Autodesk Fusion 360 part; units mm, degrees
sketch "Sketch1" plane through (0, 0, 0) normal (0, 1, 0) x (1, 0, 0)
  line L0 (0, 0) -> (0, -155)
  line L1 (-77.5, 0) -> (77.5, 0)
  line L2 (77.5, 0) -> (77.5, -155)
  line L3 (77.5, -155) -> (-77.5, -155)
  line L4 (-77.5, -155) -> (-77.5, 0)
  arc A0 (77.5, 0) -> (-77.5, 0) centre (0, 0) ccw
  line L5 (-20, -155) -> (-20, 0)
  arc A1 (20, 0) -> (-20, 0) centre (0, 0) ccw
  line L6 (20, 0) -> (20, -155)
  line L7 (-87.5, -155) -> (-87.5, 0)
  arc A2 (87.5, 0) -> (-87.5, 0) centre (0, 0) ccw
  line L8 (87.5, 0) -> (87.5, -155)
  line L9 (87.5, -155) -> (-87.5, -155)
  line L10 (-72.5, -155) -> (-72.5, 0)
  arc A3 (72.5, 0) -> (-72.5, 0) centre (0, 0) ccw
  line L11 (72.5, 0) -> (72.5, -155)
  line L12 (20, -20) -> (-20, -20)
  arc A4 (20, -20) -> (-20, -20) centre (0, -20) ccw
  dimension "d2" = 155
  dimension "d3" = 155
  dimension "d4" = 57.5
  dimension "d5" = -10
  dimension "d6" = 5
extrude "Extrude1" add sketch "Sketch1" along normal blind 7 contours L1 L3 L4 L9 L10 | L1 A0 A3 | L1 L2 L3 L9 L11
extrude "Extrude2" add sketch "Sketch1" along normal blind 3 contours L1 L5 A4 | L1 A1 | L1 L6 A4 | L1 L3 L5 L9 L10 | L1 A1 A3 | L1 L3 L6 L9 L11 | L2 L4 A0 L7 A2 L8 L9
chamfer "Chamfer1" distance 3 angle 45 3 edges at (87.5, 0, 77.5) (0, 0, -87.5) (-87.5, 0, 77.5)
equation "d2 = 245 mm - 90 mm"
equation "d4 = ( ( 155 - 40 ) / 2 ) * 1 mm"
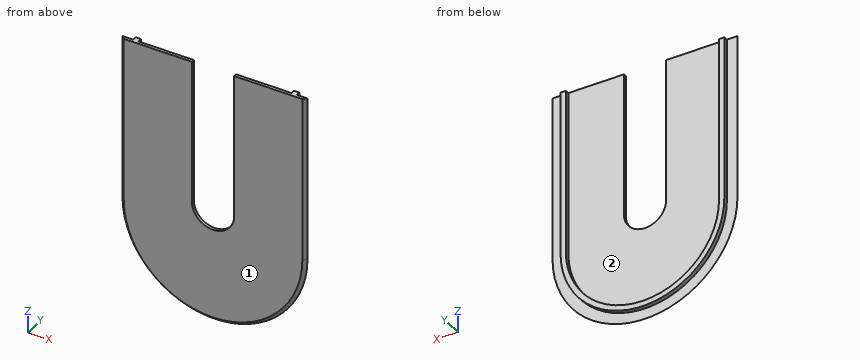
Build history of the part. All positions in model axes, mm. Face numbers are marked on the shaded views. A direction names the side the tool comes from. Give positions to 0.01 mm unless a question says otherwise; leave off trailing zeros. Loops run counter-clockwise (first coordinate to the right, second up) from the corner with the lowest first, then second, coordinate; pieces in that order, holes last.
Item 1: Slice it at C-C, the plane y = 5.25. List the corners of the cut face in (x, z).
Answers follow:
outline: (-77.5, 0) arc R77.5 ccw to (77.5, 0) - (77.5, 155) - (72.5, 155) - (72.5, 0) arc R72.5 cw to (-72.5, 0) - (-72.5, 155) - (-77.5, 155) - close
Item 2: Flat gauge pins, fed straight in: pin 1 (1.2 mm diameter, centred on y = 5, z = 46.5, fed in from -X); pin 2 (1.2 mm diameter, centred on y = 4.5, z = 55.5, fed in from +X); pin 3 (1.5 mm diameter, centred on x = -67.5, y = 1.5, fed in from -Z); pin 4 (10 mm diameter, centred on x = -14, z = 32.5, fed in from -Y). Where does each tip first touch, or does it go through?
Answers follow:
pin 1: stops at x = -77.5
pin 2: stops at x = 77.5
pin 3: stops at z = -54.81
pin 4: passes through
Item 3: Drill centre lines: line 1 (X direction, y = 5.75, z = 65.5); line 2 (Y direction, x = 52, z = 12.5); line 3 (X direction, y = 3.5, z = -21). Where is each one in solid material? Low to high.
Answers follow:
line 1: x = -77.5 to -72.5, 72.5 to 77.5
line 2: y = 0 to 3
line 3: x = -74.6 to -69.39, 69.39 to 74.6
Item 4: Which spindle directions (+Z, -Z, +X, -X, +Y, -Y) get a long thin tool onto all of the face, cutting with end or side? Do the marked faces 1 and 2. Say none if no direction does.
Answers follow:
face 1: +Z, -Z, +X, -X, -Y
face 2: +Z, +Y
